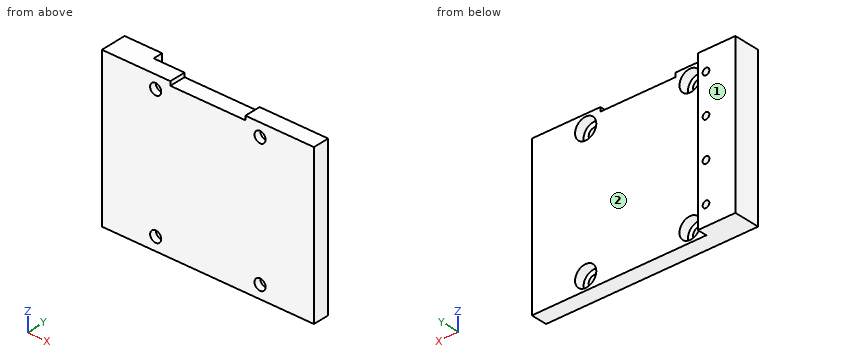
```python
from build123d import *

# Parameters (mm, degrees)
SKETCH1_W                      = 65
SKETCH1_H                      = 48
BOSS_EXTRUDE1_DEPTH            = 5
SKETCH2_W                      = 11.5
SKETCH2_H                      = 48
BOSS_EXTRUDE2_DEPTH            = 3
M2_5X0_45_TAPPED_HOLE1_D       = 2.05
M2_5X0_45_TAPPED_HOLE1_DEPTH   = 6.35
CBORE_FOR_M3_SHCS1_D           = 3.4
CBORE_FOR_M3_SHCS1_CBORE_D     = 6.5
CBORE_FOR_M3_SHCS1_CBORE_DEPTH = 3
SKETCH7_W                      = 23
SKETCH7_H                      = 5
CUT_EXTRUDE1_DEPTH             = 1.25


with BuildPart() as part:
    # Sketch1 → Boss-Extrude1 (new body)
    with BuildSketch(Plane(origin=(0, 0, 0), x_dir=(1, 0, 0), z_dir=(0, 1, 0))):
        Rectangle(SKETCH1_W, SKETCH1_H)
    extrude(amount=BOSS_EXTRUDE1_DEPTH)

    # Sketch2 → Boss-Extrude2 (add)
    with BuildSketch(Plane(origin=(0, 5, 0), x_dir=(1, 0, 0), z_dir=(0, 1, 0))):
        with Locations((-26.75, 0)):
            Rectangle(SKETCH2_W, SKETCH2_H)
    extrude(amount=BOSS_EXTRUDE2_DEPTH)

    # M2.5x0.45 Tapped Hole1
    with Locations(Plane(origin=(0, 8, 0), x_dir=(1, 0, 0), z_dir=(0, 1, 0))):
        with Locations((-23.5, 18), (-23.5, 6), (-23.5, -18), (-23.5, -6)):
            Hole(M2_5X0_45_TAPPED_HOLE1_D / 2, depth=M2_5X0_45_TAPPED_HOLE1_DEPTH)

    # CBORE for M3 SHCS1 (through all)
    with Locations(Plane(origin=(0, 5, 0), x_dir=(1, 0, 0), z_dir=(0, 1, 0))):
        with Locations((-16, 20), (16, 20), (-16, -20), (16, -20)):
            CounterBoreHole(CBORE_FOR_M3_SHCS1_D / 2, CBORE_FOR_M3_SHCS1_CBORE_D / 2, CBORE_FOR_M3_SHCS1_CBORE_DEPTH)

    # Sketch7 → Cut-Extrude1 (cut)
    with BuildSketch(Plane.XY.offset(24)):
        with Locations((0, 2.5)):
            Rectangle(SKETCH7_W, SKETCH7_H)
    extrude(amount=-CUT_EXTRUDE1_DEPTH, mode=Mode.SUBTRACT)


solid = part.part
```
The listing builds one solid part. Answer for the finished solid, in the listing's coordinates (mm). Face numbers are marked on the shaded views. A direction names the side the tool comes from. Coordinates: 2 decimals unless noted, no trailing zeros. Loops run counter-clockwise (first coordinate to the right, second up) from the corner with the lowest first, then second, coordinate; pieces in that order, holes last. Notation, with made-up numbers: (-36.75, 81) - (3.25, 81) arc R21 ccw to (3.25, 114) - close; hole circle Ø11 at (41.25, -36.5). An arc over 180 degrees is marked (long way). Use a Markdown table: item, result. Add a question column.
1) For the marked faces 1 and 2, determine the directions among +Z, -Z, +X, -X, +Y, -Y from which every point of the face is accessible in a straight line to the end or side of a thin tool.
2) Given pin 1 (2 mm diameter, centred on x = -14, z = -3.5, fed in from +Y); pin 2 (2 mm diameter, centred on x = -17.5, z = -21, fed in from +Y); pin 3 (1.6 mm diameter, centred on x = -23.5, z = -6, fed in from +Y), each flat-ended and moving along its own axis, determine where each tip first touches the part or whether it passes through.
3) The part is cut by section B-B, the plane y = 4. State how many separate pieces and enclosed holes the cut face has, and give its area (3 significant figures).
4) Find the intervals of material crossed by line 1 (Z direction, x = 16, y = 3.55); line 2 (Z direction, x = 16, y = 0.9); line 3 (X direction, y = 1.65, z = 20), in increasing order.
5) The part is cut by section C-C, the plane z = -6. Give the vertices of the cut face in (x, y) (3 decimals), and give its area (3 significant figures).
6) The part is cut by section A-A, the plane z = 20. Give the vertices of the cut face in (x, y).
7) The part is cut by section D-D, the plane x = 9. Give the vertices of the cut face in (y, z), and give its area (3 significant figures).
Here are the results:
| question | item | result |
|---|---|---|
| 1 | face 1 | +Z, -Z, +X, -X, +Y |
| 1 | face 2 | +Z, -Z, +X, +Y |
| 2 | pin 1 | stops at y = 5 |
| 2 | pin 2 | stops at y = 2 |
| 2 | pin 3 | stops at y = 1.65 |
| 3 | separate pieces | 1 |
| 3 | enclosed holes | 8 |
| 3 | area | 2,950 mm^2 |
| 4 | line 1 | z = -24 to -23.25, -16.75 to 16.75, 23.25 to 24 |
| 4 | line 2 | z = -24 to -21.7, -18.3 to 18.3, 21.7 to 24 |
| 4 | line 3 | x = -32.5 to -17.7, -14.3 to 14.3, 17.7 to 32.5 |
| 5 | outline | (-32.5, 0) - (32.5, 0) - (32.5, 5) - (-21, 5) - (-21, 8) - (-22.475, 8) - (-22.475, 1.65) - (-24.525, 1.65) - (-24.525, 8) - (-32.5, 8) - close |
| 5 | area | 346 mm^2 |
| 6 | outline | (-32.5, 0) - (-17.7, 0) - (-17.7, 2) - (-19.25, 2) - (-19.25, 5) - (-21, 5) - (-21, 8) - (-32.5, 8) - close; (-14.3, 0) - (14.3, 0) - (14.3, 2) - (12.75, 2) - (12.75, 5) - (-12.75, 5) - (-12.75, 2) - (-14.3, 2) - close; (17.7, 0) - (32.5, 0) - (32.5, 5) - (19.25, 5) - (19.25, 2) - (17.7, 2) - close |
| 7 | outline | (0, -24) - (5, -24) - (5, 22.75) - (0, 22.75) - close |
| 7 | area | 234 mm^2 |
